Can you work these out from the model? Positions are in its coordinate system, mm. A direction names the side the tool comes from. Round coordinates to 2 decimals unless told otherwise and drop trailing zeros. Loops run counter-clockwise (first coordinate to the right, second up) from the corner with the lowest first, then second, coordinate; pieces in that order, holes last. Notation, with made-up numbers: M 1.25,-32 L 53.25,-32 A19 cw 53.25,-7 Z; hole C -23,55 d11. An arc over 180 degrees is marked long. Return JSON: item names as keys, results as strings.
```python
from build123d import *

# Parameters (mm, degrees)
SKETCH005_R     = 1.7
PAD003_DEPTH    = 4
SKETCH006_W     = 8.5
SKETCH006_H     = 51
POCKET002_DEPTH = 2


with BuildPart() as part:
    # Sketch005 → Pad003 (new body)
    with BuildSketch(Plane.XY):
        with BuildLine():
            Line((35, 25.5), (-35, 25.5))
            Line((-35, 25.5), (-35, 0))
            Line((-35, 0), (-50, 0))
            Line((-50, 0), (-50, 25.5))
            ThreePointArc((-43.5, 33), (-50.5, 32.5), (-50, 25.5))
            Line((-43.5, 33), (43.5, 33))
            ThreePointArc((50, 25.5), (50.5, 32.5), (43.5, 33))
            Line((50, 0), (50, 25.5))
            Line((35, 0), (50, 0))
            Line((35, 25.5), (35, 0))
        make_face()
        with Locations((-46.75, 29.25)):
            Circle(SKETCH005_R, mode=Mode.SUBTRACT)
        with Locations((46.75, 29.25)):
            Circle(SKETCH005_R, mode=Mode.SUBTRACT)
    pad003 = extrude(amount=PAD003_DEPTH)

    # Mirrored003: Pad003 across XZ
    add(pad003.mirror(Plane.XZ))

    # Sketch006 (on Face4 of Mirrored003) → Pocket002 (cut)
    with BuildSketch(Plane(origin=(0, 0, 0), x_dir=(1, 0, 0), z_dir=(0, 0, -1))):
        with Locations((-39.25, 0)):
            Rectangle(SKETCH006_W, SKETCH006_H)
    pocket002 = extrude(amount=-POCKET002_DEPTH, mode=Mode.SUBTRACT)

    # Mirrored004: Pocket002 across Sketch006 V_Axis
    add(pocket002.mirror(Plane(origin=(0, 0, 0), x_dir=(0, 0, -1), z_dir=(1, 0, 0))), mode=Mode.SUBTRACT)


with BuildPart() as part_1:
    # Body001 placement: moved
    add(part.part.moved(Location((0, 0, 35))))


solid = part_1.part
```
Q1. If I drill on line 1 along Y through (x, z) = (46.75, 36.15); line 2 along Y through (x, z) = (20.5, 38.45); line 3 along X through (y, z) = (14, 38.15), over which ranges is the centre line in solid material (lowest first)?
Results:
{"line 1": "y = -34.21 to -30.95, -27.55 to 27.55, 30.95 to 34.21", "line 2": "y = -33 to -25.5, 25.5 to 33", "line 3": "x = -50 to -35, 35 to 50"}
Q2. Suppose I cut it at A-A, the plane z = 38.05. Please give me the cut outline in (x, y), plus the area to 3 significant figures.
Results:
{"outline": "M -50,-25.5 A4.96 ccw -43.5,-33 L 43.5,-33 A4.96 ccw 50,-25.5 L 50,25.5 A4.96 ccw 43.5,33 L -43.5,33 A4.96 ccw -50,25.5 Z; hole C -46.75,-29.25 d3.4; hole C -46.75,29.25 d3.4; hole M -35,-25.5 L 35,-25.5 L 35,25.5 L -35,25.5 Z; hole C 46.75,-29.25 d3.4; hole C 46.75,29.25 d3.4", "area": "3,050 mm2"}
Q3. On a 3-axis mill with a long thin cutter (end or side, diameter ignored), from which of +Z, -Z, +X, -X, +Y, -Y can I reach the whole of each face in a straight line? I mean faces 1 (the flat face through (-1, 33, 37)), 2 (the flat face through (-43.5, 0, 36)), 3 (the cylindrical face through (50.57, -32.42, 36.97)), 4 (the flat face through (-7, -26, 35)), 5 (the flat face through (-1, -33, 37)). Say none if no direction works.
Results:
{"face 1": "+Z, -Z, +Y", "face 2": "-Z", "face 3": "+Z, -Z", "face 4": "-Z, +X, -X, +Y, -Y", "face 5": "+Z, -Z, -Y"}
Q4. Suppose I cut it at D-D, the plane x = 10. Please give me the cut outline in (y, z).
Results:
{"outline": "M -33,35 L -25.5,35 L -25.5,39 L -33,39 Z; M 25.5,35 L 33,35 L 33,39 L 25.5,39 Z"}
Q5. Suppose I cut it at B-B, the plane y = -29.25. Please give me the cut outline in (x, z), plus the area to 4 significant figures.
Results:
{"outline": "M -51.71,35 L -48.45,35 L -48.45,39 L -51.71,39 Z; M -45.05,35 L 45.05,35 L 45.05,39 L -45.05,39 Z; M 48.45,35 L 51.71,35 L 51.71,39 L 48.45,39 Z", "area": "386.5 mm2"}
Q6. Thinking about a two-plate mould opening in X: for faces 6 (the flat face through (-50, 0, 37)), 7 (the flat face through (35, 0, 38)), 8 (the flat face through (50, 0, 37)), which applies, pulls with the +X half, pulls with the -X half, needs draft (parallel to the pull), parting line crosses it, or undercut?
Results:
{"face 6": "pulls with the -X half", "face 7": "undercut", "face 8": "pulls with the +X half"}
Q7. I'm going to push flat-ended pins straight in: pin 1 Ø1.6 at (y, z) = (11, 35.5) entering from -X; pin 2 Ø5.5 at (x, y) = (-46.75, -29.25) entering from +Z; pin 3 Ø4 at (x, y) = (-40, 7) entering from -Z; pin 4 Ø1.6 at (y, z) = (-2.5, 38) entering from +X. Where does each tip first touch, or does it pass through?
Results:
{"pin 1": "stops at x = -50", "pin 2": "stops at z = 39", "pin 3": "stops at z = 37", "pin 4": "stops at x = 50"}
Q8. Suppose I cut it at C-C, the plane x = -46.75. Please give me the cut outline in (y, z), plus the area to 3 significant figures.
Results:
{"outline": "M -34.21,35 L -30.95,35 L -30.95,39 L -34.21,39 Z; M -27.55,35 L 27.55,35 L 27.55,39 L -27.55,39 Z; M 30.95,35 L 34.21,35 L 34.21,39 L 30.95,39 Z", "area": "246 mm2"}
